from build123d import *

# Parameters (mm, degrees)
EXTRUDE_1_DEPTH   = 3
SKETCH_2_R        = 4.35
SKETCH_2_R_2      = 3.35
EXTRUDE_1_2_DEPTH = 3


with BuildPart() as part:
    # 草图1 → Extrude 1 (new body)
    with BuildSketch(Plane.XY):
        with BuildLine():
            Line((-2.478800796, 22.124879382), (-4.804808177, 4.37764987))
            ThreePointArc((-4.804808177, 4.37764987), (-6.5, 0), (-4.804808177, -4.37764987))
            Line((-4.804808177, -4.37764987), (-2.478800796, -22.124879382))
            ThreePointArc((-2.478800796, -22.124879382), (0, -24.3), (2.478800796, -22.124879382))
            Line((2.478800796, -22.124879382), (4.804808177, -4.37764987))
            ThreePointArc((4.804808177, -4.37764987), (6.5, 0), (4.804808177, 4.37764987))
            Line((4.804808177, 4.37764987), (2.478800796, 22.124879382))
            ThreePointArc((2.478800796, 22.124879382), (0, 24.3), (-2.478800796, 22.124879382))
        make_face()
    extrude(amount=EXTRUDE_1_DEPTH)

    # 草图2 → Extrude 1 2 (add)
    with BuildSketch(Plane.XY.offset(3)):
        Circle(SKETCH_2_R)
        Circle(SKETCH_2_R_2, mode=Mode.SUBTRACT)
    extrude(amount=EXTRUDE_1_2_DEPTH)


solid = part.part
CAD build for the part. Positions are in the model's coordinates, mm. A direction names the side the tool comes from. Coordinates: 2 decimals unless noted, no trailing zeros. Write each loop counter-clockwise with the first axis right and the second up, starting at its lowest first coordinate (ties: lowest second). Pieces come first, ordered by that corner, then holes. Notation, with made-up numbers: (-3, 9.5) - (55, 9.5) arc R18 ccw to (55, 23.5) - close; hole circle Ø3 at (-20.5, -17.75). An arc over 180 degrees is marked (long way). Use a Markdown table: item, result. Add a question column.
Item 1: Flat gauge pins, fed straight in: pin 1 (6 mm diameter, centred on x = 0, y = 0, fed in from +Z); pin 2 (1.5 mm diameter, centred on y = -14.5, z = 3.5, fed in from -X); pin 3 (1.5 mm diameter, centred on x = -2.5, z = 1.5, fed in from +Y). Where does each tip first touch, or does it go through?
Item 2: 3-axis set-ups, long thin cutter, end or side, ignore diameter. For faces 1 (the face through (-0.943, -4.247, 4.479)), 2 (the face through (6.5, -0.1, 1.5)): which of +Z, -Z, +X, -X, +Y, -Y reach the whole face in a straight line?
Item 3: Band-saw the part on B-B, the plane x = 0. Give the cut face in (y, z), and give its area (3 significant figures).
Item 4: Band-saw the part on A-A, the plane y = 0. Give the cut face in (x, z), and give its area (3 significant figures).
Item 5: Mould opens along Y. For faces 3 (the face through (2, -3, 6)), 4 (the face through (-3.626, 13.375, 1.479)), 5 (the face through (0, 0, 3)) say: pulls with the +Y half, pulls with the -Y half, needs draft (parallel to the pull), parting line crosses it, or undercut.
Item 6: Drill centre lines: L1, parallel to Y at x = 0, z = 3.75; L2, parallel to Z at x = -0.75, y = 2.5; L3, parallel to Y at x = 0.75, z = 1.5. Where is each one in solid material? Low to high. Write a range as from..to.
Item 7: Band-saw the part on C-C, the plane z = 4.6. Give the cut face in (x, y).
Item 8: Band-saw the part on D-D, the plane y = 12. Give the cut face in (x, z), and give its area (3 significant figures).
Numbers:
| question | item | result |
|---|---|---|
| 1 | pin 1 | z = 3 |
| 1 | pin 2 | x = -3.55 |
| 1 | pin 3 | y = 23.59 |
| 2 | face 1 | +Z |
| 2 | face 2 | +Z, -Z, +X |
| 3 | outline | (-24.3, 0) - (24.3, 0) - (24.3, 3) - (4.35, 3) - (4.35, 6) - (3.35, 6) - (3.35, 3) - (-3.35, 3) - (-3.35, 6) - (-4.35, 6) - (-4.35, 3) - (-24.3, 3) - close |
| 3 | area | 152 mm2 |
| 4 | outline | (-6.5, 0) - (6.5, 0) - (6.5, 3) - (4.35, 3) - (4.35, 6) - (3.35, 6) - (3.35, 3) - (-3.35, 3) - (-3.35, 6) - (-4.35, 6) - (-4.35, 3) - (-6.5, 3) - close |
| 4 | area | 45.0 mm2 |
| 5 | face 3 | needs draft |
| 5 | face 4 | pulls with the +Y half |
| 5 | face 5 | undercut |
| 6 | L1 | -4.35..-3.35, 3.35..4.35 |
| 6 | L2 | 0..3 |
| 6 | L3 | -24.18..24.18 |
| 7 | outline | circle Ø8.7 at (0, 0); hole circle Ø6.7 at (0, 0) |
| 8 | outline | (-3.81, 0) - (3.81, 0) - (3.81, 3) - (-3.81, 3) - close |
| 8 | area | 22.8 mm2 |
